Autodesk Fusion 360 part; units mm, degrees
sketch "スケッチ1" plane through (0, 0, 0) normal (0, 0, 1) x (1, 0, 0)
  line L0 (-3.5, 31.5) -> (3.5, 31.5)
  line L1 (3.5, 31.5) -> (17.5, 17.5)
  line L2 (17.5, 17.5) -> (17.5, -17.5)
  line L3 (17.5, -17.5) -> (3.5, -31.5)
  line L4 (3.5, -31.5) -> (-3.5, -31.5)
  line L5 (-3.5, -31.5) -> (-17.5, -17.5)
  line L6 (-17.5, -17.5) -> (-17.5, 17.5)
  line L7 (-17.5, 17.5) -> (-3.5, 31.5)
  circle A0 centre (-12.5, 12.5) radius 3
  circle A1 centre (-12.5, -12.5) radius 3
  circle A2 centre (12.5, -12.5) radius 3
  circle A3 centre (12.5, 12.5) radius 3
  dimension "d1" = 35
  dimension "d2" = 63
  dimension "d3" = 31.5
  dimension "d4" = 17.5
  dimension "d5" = 14
  dimension "d6" = 14
  dimension "d7" = 14
  dimension "d8" = 14
  dimension "d9" = 14
  dimension "d10" = 14
  dimension "d11" = 14
  dimension "d12" = 14
  dimension "d13" = 6
  dimension "d14" = 12.5
  dimension "d15" = 12.5
  dimension "d17" = 360
extrude "押し出し1" add sketch "スケッチ1" along normal blind 12.5 contours L0 L1 L2 L3 L4 L5 L6 L7 | A0 | A1 | A2 | A3
extrude "押し出し2" cut sketch "スケッチ1" along normal blind 3 contours A0 | A1 | A2 | A3
sketch "スケッチ2" plane through (17.5, 0, 0) normal (1, 0, 0) x (0, 1, 0)
  line L0 (-17.5, 0) -> (17.5, 0)
  line L1 (17.5, 0) -> (17.5, 12.5)
  line L2 (17.5, 12.5) -> (-17.5, 12.5)
  line L3 (-17.5, 12.5) -> (-17.5, 0)
  circle A0 centre (0, 12.75) radius 9.5
  line L4 (17.5, 0) -> (-17.5, 0)
  dimension "d22" = 19
  dimension "d23" = 12.75
extrude "押し出し3" cut sketch "スケッチ2" against normal up to surface (35 mm away) contours L2 A0 picked at (1.5592, 9.8271)
sketch "スケッチ3" plane through (0, 0, 12.5) normal (0, 0, 1) x (-1, 0, 0)
  line L0 (17.5, -9.4967) -> (-17.5, -9.4967)
  line L1 (-17.5, -9.4967) -> (-17.5, -17.5)
  line L2 (-17.5, -17.5) -> (-3.5, -31.5)
  line L3 (-3.5, -31.5) -> (3.5, -31.5)
  line L4 (3.5, -31.5) -> (17.5, -17.5)
  line L5 (17.5, -17.5) -> (17.5, -9.4967)
  circle A0 centre (12.5, -12.5) radius 1.75
  circle A1 centre (12.5, 12.5) radius 1.75
  circle A2 centre (-12.5, 12.5) radius 1.75
  circle A3 centre (-12.5, -12.5) radius 1.75
  line L6 (-3.5, 31.5) -> (3.5, 31.5)
  line L7 (0, 31.5) -> (0, -31.5) construction
  circle A4 centre (0, 22.5) radius 5.5
  circle A5 centre (0, -22.5) radius 5.5
  point P0 (12.5, -12.5)
  dimension "d26" = 3.5
  dimension "d28" = 360
  dimension "d32" = 11
  dimension "d33" = 11
  dimension "d34" = 9
  dimension "d35" = 9
extrude "押し出し4" cut sketch "スケッチ3" against normal blind 9.1 contours A0 | A1 | A2 | A3
extrude "押し出し5" cut sketch "スケッチ3" against normal blind 5 contours A4 | A5
fillet "フィレット1" radius 5 8 edges at (-17.5, 17.5, 6.25) (-3.5, 31.5, 6.25) (3.5, 31.5, 6.25) (17.5, 17.5, 6.25) (-17.5, -17.5, 6.25) (-3.5, -31.5, 6.25) (3.5, -31.5, 6.25) (17.5, -17.5, 6.25)
equation "d3 = d2 / 2"
equation "d4 = d1 / 2"
equation "d7 = d5"
equation "d8 = d6"
equation "d9 = d5"
equation "d10 = d7"
equation "d11 = d10"
equation "d12 = d9"
Model file for the job. Use its own axes, mm. A direction names the side the tool comes from. Round coordinates to 2 decimals unless told otherwise and drop trailing zeros. Write each loop counter-clockwise with the first axis right and the second up, starting at its lowest first coordinate (ties: lowest second). Pieces come first, ordered by that corner, then holes. Notation, with made-up numbers: (-5, -11.75) - (10, -11.75) arc R36 cw to (10, 22.25) - close; hole circle Ø5 at (-14, -1). An arc over 180 degrees is marked (long way). Use CSV: the item, a comma, the result in double quotes. Start each with the question number.
Item 1: Two-plate mould, pull along X, no slides. Class faces 4 (the face through (3.32, -31.13, 6.34)), 5 (the face through (13, -13, 3.4)), 6 (the face through (-10, -25, 6)): released by +X, released by -X, zero draft, split by the parting line, or undercut.
Item 2: Band-saw the part on A-A (z = 10). Write the cut outline in (x, y).
Item 3: Band-saw the part on C-C (y = -22.5). Write the cut outline in (x, z), and give its area (4 significant figures).
Item 4: Band-saw the part on D-D (y = 0). Write the cut outline in (x, z), and give its area (3 significant figures).
Item 5: Pin check, flat tips, straight feed: P1, Ø12, axis at x = -1, y = 22, coming from the +Z side; P2, Ø1, axis at x = 12.5, y = 13, coming from the +Z side; P3, Ø3, axis at x = 12.5, y = -12.5, coming from the -Z side; P4, Ø2, axis at x = 3, y = -23, coming from the +Z side. Stop position of each tip, or through.
Item 6: Drill centre lines: L1, parallel to X at y = 12.5, z = 6.75; L2, parallel to Y at x = 11, z = 10; L3, parallel to Y at x = -12.5, z = 9.25. Where is each one in solid material? Low to high. Write a range as [from, to].
Item 7: Tool access for faces 1 (the face through (-3.37, -31.11, 6.34)), 2 (the face through (-12, 12, 3.4)), 3 (the face through (-13, 13, 3)): list every direction of +Z, -Z, +X, -X, +Y, -Y with a clear straight run to the whole face (end or side of a thin tool).
Checked values:
1,face 4,"released by +X"
1,face 5,"undercut"
1,face 6,"released by -X"
2,outline,"(-17.5, -15.43) arc R5 ccw to (-16.04, -18.96) - (-4.96, -30.04) arc R5 ccw to (-1.43, -31.5) - (1.43, -31.5) arc R5 ccw to (4.96, -30.04) - (16.04, -18.96) arc R5 ccw to (17.5, -15.43) - (17.5, -9.09) - (-17.5, -9.09) - close; (-17.5, 9.09) - (17.5, 9.09) - (17.5, 15.43) arc R5 ccw to (16.04, 18.96) - (4.96, 30.04) arc R5 ccw to (1.43, 31.5) - (-1.43, 31.5) arc R5 ccw to (-4.96, 30.04) - (-16.04, 18.96) arc R5 ccw to (-17.5, 15.43) - close; hole circle Ø3.5 at (-12.5, -12.5); hole circle Ø3.5 at (-12.5, 12.5); hole circle Ø11 at (0, -22.5); hole circle Ø11 at (0, 22.5); hole circle Ø3.5 at (12.5, -12.5); hole circle Ø3.5 at (12.5, 12.5)"
3,outline,"(-12.5, 0) - (12.5, 0) - (12.5, 12.5) - (5.5, 12.5) - (5.5, 7.5) - (-5.5, 7.5) - (-5.5, 12.5) - (-12.5, 12.5) - close"
3,area,"257.5 mm²"
4,outline,"(-17.5, 0) - (17.5, 0) - (17.5, 3.25) - (-17.5, 3.25) - close"
4,area,"114 mm²"
5,P1,"stops at z = 12.5"
5,P2,"stops at z = 3.4"
5,P3,"stops at z = 3"
5,P4,"stops at z = 7.5"
6,L1,"x = [-17.5, -14.25], [-10.75, 10.75], [14.25, 17.5]"
6,L2,"y = [-24, -13.4], [-11.6, -9.09], [9.09, 11.6], [13.4, 24]"
6,L3,"y = [-22.5, -14.25], [-10.75, -8.83], [8.83, 10.75], [14.25, 22.5]"
7,face 1,"+Z, -Z, -X, -Y"
7,face 2,"+Z"
7,face 3,"-Z"
